```python
from build123d import *

# Parameters (mm, degrees)
EXTRUDE_1_DEPTH         = 30
HOLE_WIZARD_4_2_4_2_1_D = 4.2
SKETCH_7_R              = 5
CUT_EXTRUDE_1_DEPTH     = 20


with BuildPart() as part:
    # 草图1 → 凸台-拉伸1 (new body)
    with BuildSketch(Plane.XY):
        with BuildLine():
            Line((-27.342107977, 47.722207948), (3.772223289, 31.776883602))
            ThreePointArc((3.772223289, 31.776883602), (30.070163865, 10.944644586), (23.315477742, -21.917766712))
            Line((23.315477742, -21.917766712), (9.729974097, -54.132500442))
            ThreePointArc((9.729974097, -54.132500442), (51.683094143, 18.811107883), (-27.342107977, 47.722207948))
        make_face()
    extrude(amount=EXTRUDE_1_DEPTH)

    # Ø4.2 (4.2) 直径孔1 (through all)
    with Locations(Plane(origin=(0, 42, 30), x_dir=(1, 0, 0), z_dir=(0, 0, 1))):
        with Locations((0, 0), (29.69848481, -12.30151519), (42, -42), (29.69848481, -71.69848481)):
            Hole(HOLE_WIZARD_4_2_4_2_1_D / 2)

    # 草图7 → 切除-拉伸1 (cut)
    with BuildSketch(Plane(origin=(0, 0, 0), x_dir=(-1, 0, 0), z_dir=(0, 0, -1))):
        with Locations((0, 42)):
            Circle(SKETCH_7_R)
        with Locations((-29.69848481, 29.69848481)):
            Circle(SKETCH_7_R)
        with Locations((-42, 0)):
            Circle(SKETCH_7_R)
        with Locations((-29.69848481, -29.69848481)):
            Circle(SKETCH_7_R)
    extrude(amount=-CUT_EXTRUDE_1_DEPTH, mode=Mode.SUBTRACT)


solid = part.part
```
Model file for the job. Use its own axes, mm. A direction names the side the tool comes from. Coordinates: 2 decimals unless noted, no trailing zeros. Loops run counter-clockwise (first coordinate to the right, second up) from the corner with the lowest first, then second, coordinate; pieces in that order, holes last. Notation, with made-up numbers: (-30.75, 18) - (7.25, 18) arc R27 ccw to (7.25, 49) - close; hole circle Ø5 at (0, 42). An arc over 180 degrees is marked (long way). Write item = value, one per line. Start each with the question number.
Item 1: Drop flat-ended pins along their axis: pin 1 Ø4 at (x, y) = (0, 42) entering from -Z; pin 2 Ø9 at (x, y) = (0, 42) entering from -Z; pin 3 Ø3 at (y, z) = (3, 9.5) entering from +X; pin 4 Ø1 at (x, z) = (31.5, 18.5) entering from -Y. Give the stop position or say it passes through.
Item 2: Pull direction X, two halves, no side cores. Call faces 1 (the face through (33.7, 26.7, 9.9)), 2 (the face through (29.9, 11.4, 14.8)), 3 (the face through (32, 13, 30)): +X half, -X half, draft (parallel to the pull), parting line (faces both ways), or undercut.
Item 3: Saw through at A-A, the plane y = 0. List the corners of the cut face in (x, z), then the cut area to 3 significant figures.
Item 4: Saw through at C-C, the plane z = 7.5. List the corners of the cut face in (x, y).
Item 5: Saw through at D-D, the plane x = 17.5. List the corners of the cut face in (y, z), then the cut area to 3 significant figures.
Item 6: Saw through at B-B, the plane x = 42. List the corners of the cut face in (y, z), then the cut area to 3 significant figures.
Item 7: 3-axis set-ups, long thin cutter, end or side, ignore diameter. For faces 4 (the face through (0.651, 46.957, 9.86)), 5 (the face through (16.618, -37.8, 14.79)), 6 (the face through (-12, 39.86, 14.79)): which of +Z, -Z, +X, -X, +Y, -Y reach the whole face in a straight line?
Item 8: Wall check: probe 1 along Y at (x, z) = (28.5, 5); probe 2 along Y at (x, z) = (33.5, 8.75); probe 3 along X at (y, z) = (1, 23). Give the ranges that are in metal, low to high. Write a range as [from, to].
Answers:
q1.pin_1 = through
q1.pin_2 = 20
q1.pin_3 = 54.98
q1.pin_4 = -45.43
q2.face_1 = undercut
q2.face_2 = -X half
q2.face_3 = draft
q3.outline = (32, 0) - (37, 0) - (37, 20) - (39.9, 20) - (39.9, 30) - (32, 30) - close; (44.1, 20) - (47, 20) - (47, 0) - (55, 0) - (55, 30) - (44.1, 30) - close
q3.area = 448 mm2
q4.outline = (-27.34, 47.72) - (3.77, 31.78) arc R32 cw to (23.32, -21.92) - (9.73, -54.13) arc R55 ccw (long way) to start; hole circle Ø10 at (0, 42); hole circle Ø10 at (29.7, -29.7); hole circle Ø10 at (29.7, 29.7); hole circle Ø10 at (42, 0)
q5.outline = (-52.14, 0) - (-35.71, 0) - (-35.71, 30) - (-52.14, 30) - close; (26.79, 0) - (52.14, 0) - (52.14, 30) - (26.79, 30) - close
q5.area = 1,250 mm2
q6.outline = (-35.51, 0) - (-5, 0) - (-5, 20) - (-2.1, 20) - (-2.1, 30) - (-35.51, 30) - close; (2.1, 20) - (5, 20) - (5, 0) - (35.51, 0) - (35.51, 30) - (2.1, 30) - close
q6.area = 1,890 mm2
q7.face_4 = -Z
q7.face_5 = +Z, -Z, -X
q7.face_6 = +Z, -Z, -X, -Y
q8.probe_1 = [-47.04, -34.55], [-24.84, -14.55], [14.55, 24.84], [34.55, 47.04]
q8.probe_2 = [-43.62, -32.95], [-26.45, 26.45], [32.95, 43.62]
q8.probe_3 = [31.98, 40.15], [43.85, 54.99]
